from build123d import *

# Parameters (mm, degrees)
SKETCH1_R           = 1.219603507
BOSS_EXTRUDE1_DEPTH = 1.6256
SKETCH2_W           = 8.4963
SKETCH2_H           = 8.5725
BOSS_EXTRUDE2_DEPTH = 4.572


with BuildPart() as part:
    # Sketch1 → Boss-Extrude1 (new body)
    with BuildSketch(Plane.XY):
        with BuildLine():
            Line((-11.39825, -17.8054), (11.39825, -17.8054))
            Line((11.39825, -17.8054), (11.39825, 16.4084))
            ThreePointArc((11.39825, 16.4084), (10.989078173, 17.396228173), (10.00125, 17.8054))
            Line((10.00125, 17.8054), (-10.00125, 17.8054))
            ThreePointArc((-10.00125, 17.8054), (-10.989078173, 17.396228173), (-11.39825, 16.4084))
            Line((-11.39825, 16.4084), (-11.39825, -17.8054))
        make_face()
        with Locations((-10.00125, 16.4084)):
            Circle(SKETCH1_R, mode=Mode.SUBTRACT)
        with Locations((10.00125, 16.4084)):
            Circle(SKETCH1_R, mode=Mode.SUBTRACT)
    extrude(amount=BOSS_EXTRUDE1_DEPTH)

    # Sketch2 → Boss-Extrude2 (add)
    with BuildSketch(Plane.XY.offset(1.6256)):
        with Locations((0.1905, 13.2334)):
            Rectangle(SKETCH2_W, SKETCH2_H)
    extrude(amount=BOSS_EXTRUDE2_DEPTH)


solid = part.part
The model under review builds one solid part; all positions refer to its coordinate system, in mm. A direction names the side the tool comes from. Give positions to 0.01 mm unless a question says otherwise; leave off trailing zeros. Write each loop counter-clockwise with the first axis right and the second up, starting at its lowest first coordinate (ties: lowest second). Pieces come first, ordered by that corner, then holes. Notation, with made-up numbers: M -8.5,31 L 16.5,31 A14 ccw 16.5,53 Z; hole C 19,17 d9. An arc over 180 degrees is marked long. One line per question, with ' | ' between items. Start each with the question number.
Item 1: We need section D-D on y = -8. Write out the cut boundary in (x, z).
Item 2: We need section C-C on z = 3.25. Write out the cut boundary in (x, y), plus the area to 3 significant figures.
Item 3: For faces 5 (the flat face through (0, 17.52, 4)), 6 (the flat face through (0, 8.947, 4)), 7 (the flat face through (-4.058, 13, 4)), list the 3-axis set-ups (+Z, -Z, +X, -X, +Y, -Y) from which the entire face can be reached by the end or side of a thin tool; tool diameter is ignored.
Item 4: We need section A-A on y = 11.5. Write out the cut boundary in (x, z), plus the area to 3 significant figures.
Item 5: For pin 1 (2.5 mm diameter, centred on x = 1, z = 3.5, fed in from +Y); pin 2 (4 mm diameter, centred on x = 6, y = 0, fed in from +Z); pin 3 (3.5 mm diameter, centred on y = 13, z = 5, fed in from -X), all flat-tipped, find the tip position at first contact; note any pin that passes through.
Item 6: Draft analysis for pull direction Y (two halves, no side actions). For faces 1 (the flat face through (-11.398, 0, 1)), 2 (the cylindrical face through (-9.438, 15.326, 0.801)), 3 (the cylindrical face through (9.737, 15.218, 0.801)), 4 (the flat face through (0, -17.805, 1)), state which applies: released by +Y, released by -Y, zero draft, split by the parting line, or undercut.
Item 7: We need section B-B on x = 0.5. Write out the cut boundary in (y, z).
Item 8: Wall thickness on line 1 (Y direction, x = 10, z = 1); line 2 (X direction, y = 16.5, z = 3.75); line 3 (Y direction, x = -0.5, z = 3): over which ranges is each line inside the solid? List them lowest first. Write a range as from..to.
Results found:
1) outline: M -11.4,0 L 11.4,0 L 11.4,1.63 L -11.4,1.63 Z
2) outline: M -4.06,8.95 L 4.44,8.95 L 4.44,17.52 L -4.06,17.52 Z | area: 72.8 mm2
3) face 5: +Z, +X, -X, +Y | face 6: +Z, +X, -X, -Y | face 7: +Z, -X, +Y, -Y
4) outline: M -11.4,0 L 11.4,0 L 11.4,1.63 L 4.44,1.63 L 4.44,6.2 L -4.06,6.2 L -4.06,1.63 L -11.4,1.63 Z | area: 75.9 mm2
5) pin 1: stops at y = 17.52 | pin 2: stops at z = 1.63 | pin 3: stops at x = -4.06
6) face 1: zero draft | face 2: undercut | face 3: undercut | face 4: released by -Y
7) outline: M -17.81,0 L 17.81,0 L 17.81,1.63 L 17.52,1.63 L 17.52,6.2 L 8.95,6.2 L 8.95,1.63 L -17.81,1.63 Z
8) line 1: y = -17.81..15.19, 17.63..17.81 | line 2: x = -4.06..4.44 | line 3: y = 8.95..17.52
